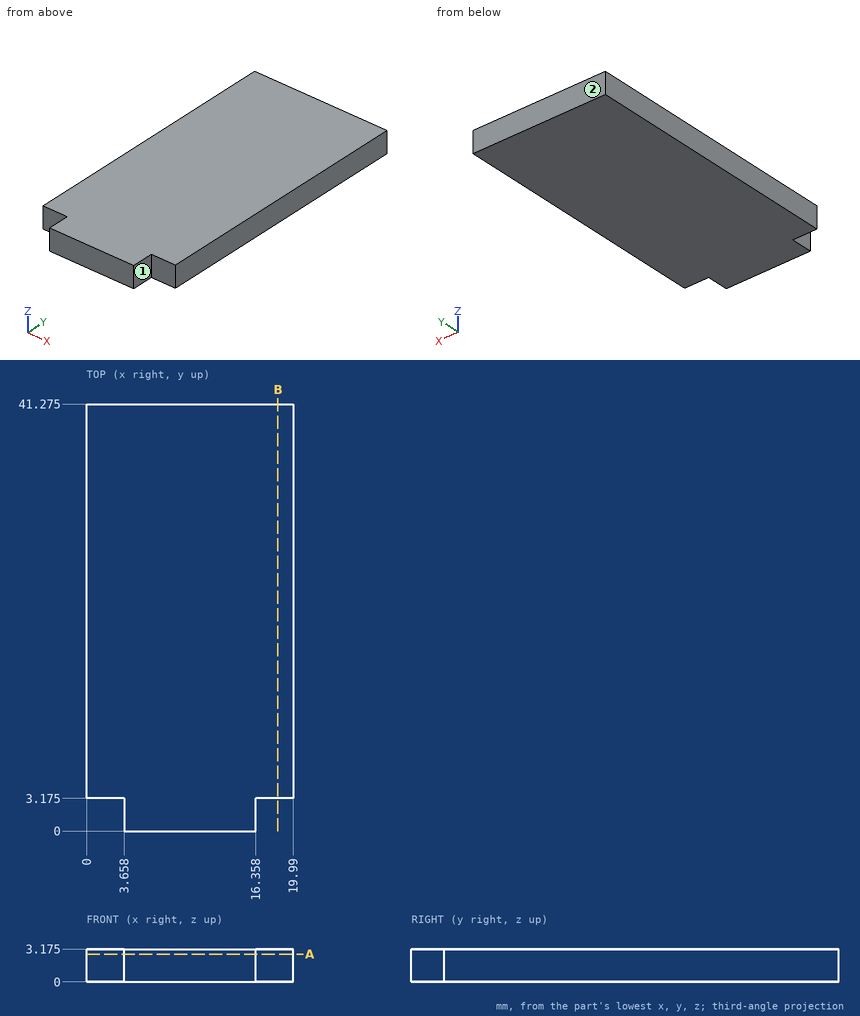
Geometry check sheet. Reference: drawing and pictorial views, mm from the part's lowest x, y, z. A direction names the side the tool comes from. Round coordinates to 2 decimals unless told otherwise and drop trailing zeros. Order: outer loops, then holes, each group sorted by start corner. A loop starts at its lowest first (then second) coordinate and runs counter-clockwise, first axis right, second up. Notation, with made-up numbers: (25.25, -12) -> (37.25, -12) arc R9 ccw to (37.25, 3) -> close; hole circle Ø9 at (3, 25.5). An arc over 180 degrees is marked (long way). One line per item, written item: value. Start each with the question number.
Q1. Cross-section at A-A (z = 2.7). Record the boundary of the cut face in (x, y) (1 decimal), and give its area (3 significant figures).
Q2. Cross-section at B-B (x = 18.5). Record the boundary of the cut face in (y, z) (1 decimal).
Q3. Gauge pin test, flat ends, axial feed: pin 1 Ø1 at (y, z) = (1, 1.5) entering from +X; pin 2 Ø1 at (x, z) = (17.5, 1) entering from -Y (3 decimals); pin 3 Ø1.6 at (y, z) = (2, 2) entering from -X. Record the tip position at first contact, or that the pin passes through.
Q4. Thickness scan on line 1 (Y direction, x = 2.75, z = 0.5) (1 decimal). Record the ranges inside material, lowest first.
Q5. Set-up check for the marked faces 1 and 2: record each of +Z, -Z, +X, -X, +Y, -Y from which the full face is reachable in a straight line by a thin tool's end or side.
Completed:
1. outline: (0, 3.2) -> (3.7, 3.2) -> (3.7, 0) -> (16.4, 0) -> (16.4, 3.2) -> (20, 3.2) -> (20, 41.3) -> (0, 41.3) -> close
1. area: 802 mm²
2. outline: (3.2, 0) -> (41.3, 0) -> (41.3, 3.2) -> (3.2, 3.2) -> close
3. pin 1: stops at x = 16.36
3. pin 2: stops at y = 3.175
3. pin 3: stops at x = 3.66
4. line 1: y = 3.2 to 41.3
5. face 1: +Z, -Z, +X, -Y
5. face 2: +Z, -Z, +X, -X, +Y
